The listing builds one solid part. Answer for the finished solid, in the listing's coordinates (mm). A direction names the side the tool comes from. Give positions to 0.01 mm unless a question says otherwise; leave off trailing zeros. Write each loop counter-clockwise with the first axis right and the second up, starting at its lowest first coordinate (ties: lowest second). Pieces come first, ordered by that corner, then holes. Notation, with made-up numbers: (-37, -37.75) - (16, -37.75) arc R4 ccw to (16, -30.75) - close; hole circle Ø3 at (76.5, -17). An arc over 180 degrees is marked (long way). Write each question's results on one line, items separated by ' | '. Start each with the question number.
Q1. Find the intervals of material crossed by probe 1 along Y at (x, z) = (-12, 1.4); probe 2 along X at (y, z) = (4.25, 0.95); probe 3 along Z at (x, y) = (0.5, -7), in increasing order.
Q2. For a pull along Y with two mould halves and no side action, classify faces 5 (the face through (0, 12.6, 1)), 6 (the face through (3, 0, 0)), 7 (the face through (13.016, -7.421, 1.521)) as pulls with the +Y half, pulls with the -Y half, needs draft (parallel to the pull), parting line crosses it, or undercut.
Q3. Flat-ended cylindrical pins translate along their axes: pin 1 Ø2.5 at (y, z) = (-1, 1) entering from -X; pin 2 Ø2.5 at (x, z) = (-11, 1) entering from +Y; pin 3 Ø2.5 at (y, z) = (-11.5, 1.5) entering from +X; pin 4 Ø3 at (y, z) = (6, 2.5) entering from -X. Find the tip coordinate at first contact, or state that the pin passes through.
Q4. Section D-D (y = 0) is taken. Determine the outline of the cut face in (x, z), plus the area to 4 significant figures.
Q5. Section B-B (z = 1.65) is taken. Determine the outline of the cut face in (x, y), plus the area to 3 significant figures.
Q6. Section A-A (y = -7) is taken. Determine the outline of the cut face in (x, z), plus the area to 3 significant figures.
Q7. Section C-C (x = -0.5) is taken. Determine the outline of the cut face in (y, z).
Q8. For faces 1 (the face through (11, 9.25, 2)), 2 (the face through (-9.6, -11, 1)), 3 (the face through (-11, 4.75, 2)), 4 (the face through (-2.6, 0, 0.4)), determine the directions among +Z, -Z, +X, -X, +Y, -Y from which every point of the face is accessible in a straight line to the end or side of a thin tool.
```python
from build123d import *

# Parameters (mm, degrees)
SKETCH_1_W          = 19.2
SKETCH_1_H          = 25.2
EXTRUDE_1_DEPTH     = 3
SKETCH_3_R          = 1.1
EXTRUDE_2_DEPTH     = 3
SKETCH_4_R          = 1.15
CUT_EXTRUDE_1_DEPTH = 7
SKETCH_5_R          = 2.5
EXTRUDE_3_DEPTH     = 3


with BuildPart() as part:
    # 草图1 → 凸台-拉伸1 (new body)
    with BuildSketch(Plane.XY):
        Rectangle(SKETCH_1_W, SKETCH_1_H)
    extrude(amount=EXTRUDE_1_DEPTH)

    # 草图3 → 凸台-拉伸2 (add, through all)
    with BuildSketch(Plane.XY.offset(3)):
        with BuildLine():
            Line((12, 9.25), (9.6, 9.25))
            Line((9.6, 9.25), (9.6, 4.75))
            Line((9.6, 4.75), (12, 4.75))
            ThreePointArc((12, 4.75), (14.25, 7), (12, 9.25))
        make_face()
        with Locations((12, 7)):
            Circle(SKETCH_3_R, mode=Mode.SUBTRACT)
        with BuildLine():
            Line((9.6, -9.25), (9.6, -4.75))
            Line((9.6, -4.75), (12, -4.75))
            ThreePointArc((12, -4.75), (14.25, -7), (12, -9.25))
            Line((12, -9.25), (9.6, -9.25))
        make_face()
        with Locations((12, -7)):
            Circle(SKETCH_3_R, mode=Mode.SUBTRACT)
        with BuildLine():
            Line((-12, -9.25), (-9.6, -9.25))
            Line((-9.6, -9.25), (-9.6, -4.75))
            Line((-9.6, -4.75), (-12, -4.75))
            ThreePointArc((-12, -4.75), (-14.25, -7), (-12, -9.25))
        make_face()
        with Locations((-12, -7)):
            Circle(SKETCH_3_R, mode=Mode.SUBTRACT)
        with BuildLine():
            Line((-9.6, 9.25), (-9.6, 4.75))
            Line((-9.6, 4.75), (-12, 4.75))
            ThreePointArc((-12, 4.75), (-14.25, 7), (-12, 9.25))
            Line((-12, 9.25), (-9.6, 9.25))
        make_face()
        with Locations((-12, 7)):
            Circle(SKETCH_3_R, mode=Mode.SUBTRACT)
    extrude_2 = extrude(amount=-EXTRUDE_2_DEPTH)

    # 镜向1: 凸台-拉伸2 across plane
    add(extrude_2.mirror(Plane.ZX))

    # 草图4 → 切除-拉伸1 (cut)
    with BuildSketch(Plane(origin=(-9.6, 3, 0), x_dir=(0, 1, 0), z_dir=(-1, 0, 0))):
        with Locations((-3, 0)):
            Circle(SKETCH_4_R)
    extrude(amount=-CUT_EXTRUDE_1_DEPTH, mode=Mode.SUBTRACT)

    # 草图5 → 凸台-拉伸3 (add)
    with BuildSketch(Plane(origin=(0, 0, 0), x_dir=(-1, 0, 0), z_dir=(0, 0, -1))):
        Circle(SKETCH_5_R)
    extrude(amount=EXTRUDE_3_DEPTH)


solid = part.part
```
Answers below:
1) probe 1: y = -9.25 to -8.1, -5.9 to -4.75, 4.75 to 5.9, 8.1 to 9.25 | probe 2: x = -9.6 to 9.6 | probe 3: z = 0 to 3
2) face 5: pulls with the +Y half | face 6: needs draft | face 7: undercut
3) pin 1: stops at x = -9.6 | pin 2: stops at y = 9.25 | pin 3: stops at x = 9.6 | pin 4: stops at x = -14.25
4) outline: (-9.6, 1.15) - (-2.6, 1.15) - (-2.6, 0) - (-2.5, 0) - (-2.5, -3) - (2.5, -3) - (2.5, 0) - (9.6, 0) - (9.6, 3) - (-9.6, 3) - close | area: 64.55 mm2
5) outline: (-12, -9.25) - (-9.6, -9.25) - (-9.6, -12.6) - (9.6, -12.6) - (9.6, -9.25) - (12, -9.25) arc R2.25 ccw to (12, -4.75) - (9.6, -4.75) - (9.6, 4.75) - (12, 4.75) arc R2.25 ccw to (12, 9.25) - (9.6, 9.25) - (9.6, 12.6) - (-9.6, 12.6) - (-9.6, 9.25) - (-12, 9.25) arc R2.25 ccw to (-12, 4.75) - (-9.6, 4.75) - (-9.6, -4.75) - (-12, -4.75) arc R2.25 ccw to start; hole circle Ø2.2 at (-12, -7); hole circle Ø2.2 at (-12, 7); hole circle Ø2.2 at (12, -7); hole circle Ø2.2 at (12, 7) | area: 544 mm2
6) outline: (-14.25, 0) - (-13.1, 0) - (-13.1, 3) - (-14.25, 3) - close; (-10.9, 0) - (10.9, 0) - (10.9, 3) - (-10.9, 3) - close; (13.1, 0) - (14.25, 0) - (14.25, 3) - (13.1, 3) - close | area: 72.3 mm2
7) outline: (-12.6, 0) - (-2.45, 0) - (-2.45, -3) - (2.45, -3) - (2.45, 0) - (12.6, 0) - (12.6, 3) - (-12.6, 3) - close
8) face 1: +Z, -Z, +X, +Y | face 2: +Z, -Z, -X, -Y | face 3: +Z, -Z, -X | face 4: -Z, -X
